The figure shows three views and two pictorial views of one solid part (mm, origin at its lowest corner). Answer the questions. Coordinates: 2 decimals unless noted, no trailing zeros. Write each loop counter-clockwise with the first axis right and the second up, starting at its lowest first coordinate (ties: lowest second). Pieces come first, ordered by that corner, then holes.
Item 1: Section B-B (y = 40) is taken. Give the vertices of the cut face in (x, z) (1 decimal), then the cut area to 3 significant figures.
Item 2: Section C-C (z = 23.5) is taken. Give the vertices of the cut face in (x, y) (1 decimal), then the cut area to 3 significant figures.
Item 3: Straight lines are drawn through the part: probe 1 along Z at (x, y) = (19.5, 47.5) (1 decimal); probe 2 along Y at (x, z) = (20, 28) (1 decimal); probe 3 along Y at (x, z) = (11, 23) (1 decimal). For each, find the intervals that lie inside material, in ascending order.
Item 4: Each of these flat-tipped pins is pushed along its axis until it touches: P1, Ø5, axis at x = 11, z = 34, coming from the -Y side; P2, Ø5, axis at x = 8, z = 11, coming from the -Y side; P3, Ø3, axis at x = 19, z = 29, coming from the +Y side. Where does it stop, or does it pass through?
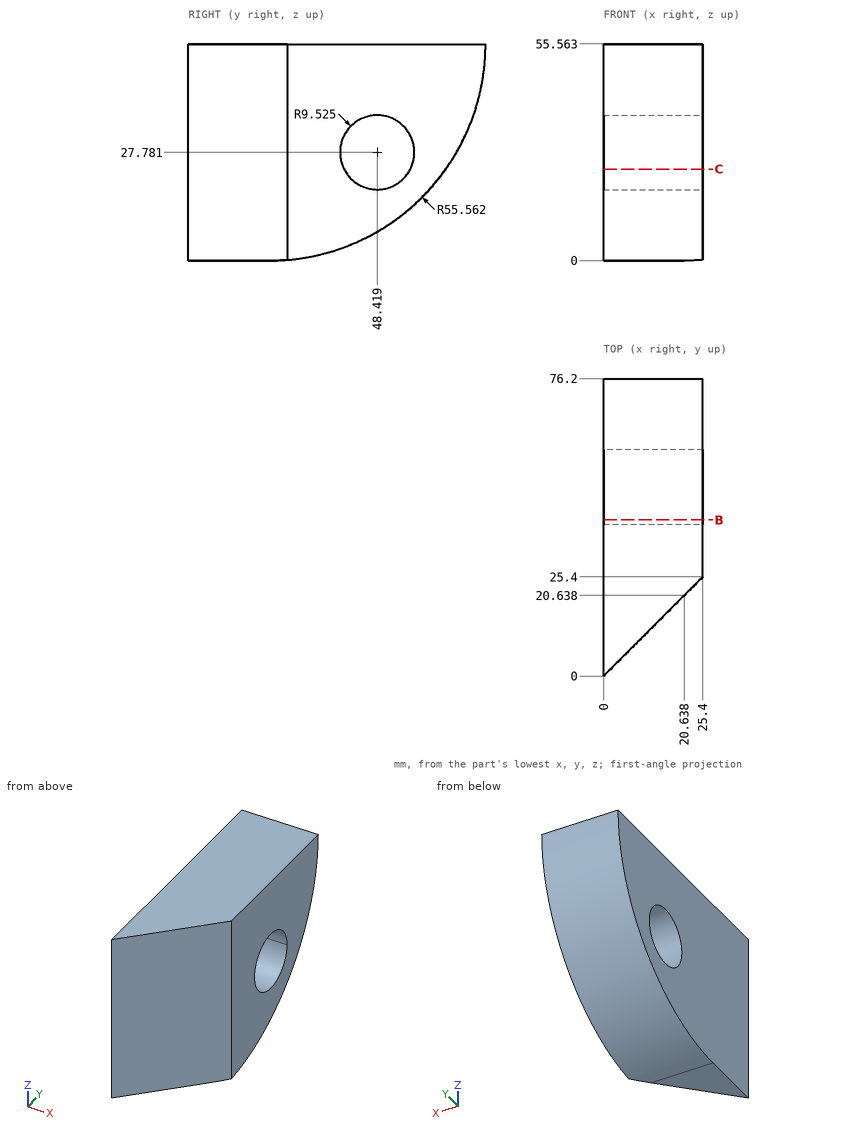
Established:
1. outline: (0, 3.5) - (25.4, 3.5) - (25.4, 23.3) - (0, 23.3) - close; (0, 32.2) - (25.4, 32.2) - (25.4, 55.6) - (0, 55.6) - close
1. area: 1,100 mm2
2. outline: (0, 0) - (25.4, 25.4) - (25.4, 39.9) - (0, 39.9) - close; (0, 56.9) - (25.4, 56.9) - (25.4, 66) - (0, 66) - close
2. area: 922 mm2
3. probe 1: z = 6.9 to 18.3, 37.3 to 55.6
3. probe 2: y = 20 to 38.9, 57.9 to 68.9
3. probe 3: y = 11 to 40.2, 56.7 to 65.7
4. P1: stops at y = 8.5
4. P2: stops at y = 5.5
4. P3: stops at y = 70.23
